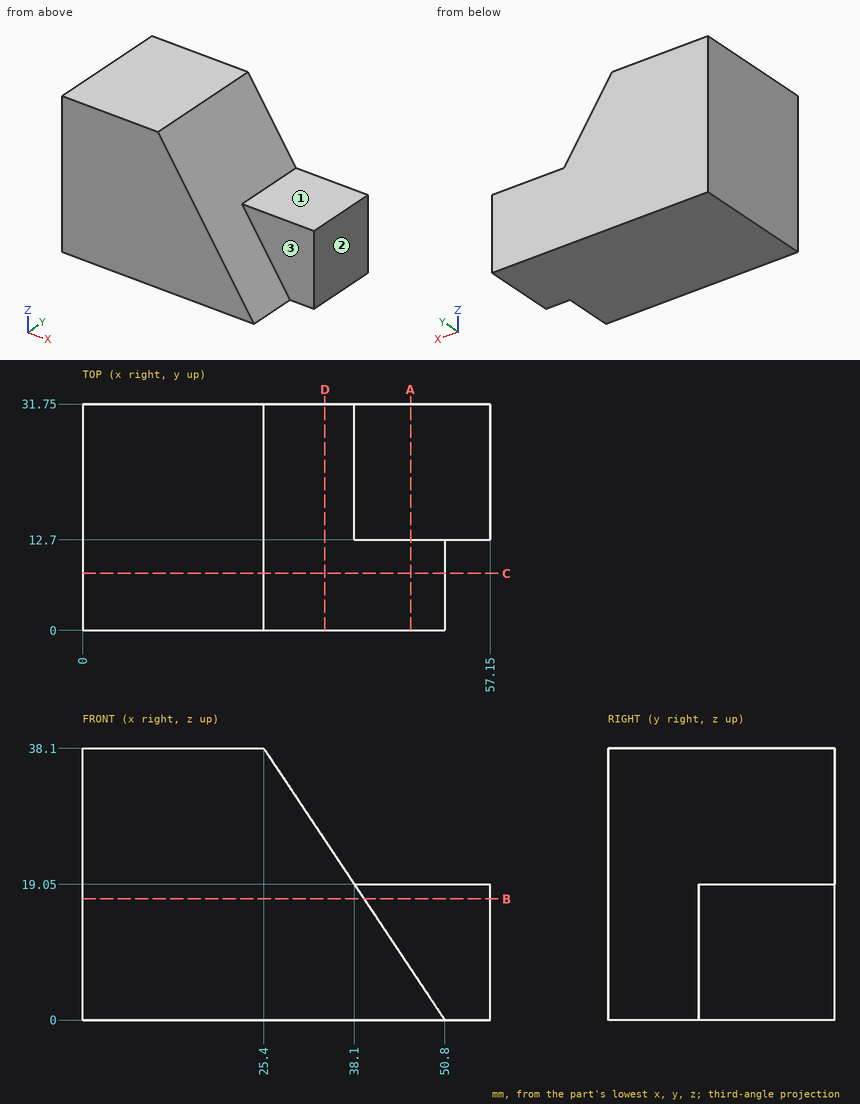
Here's the drawing with two shaded views (mm, measured from the low corner). I have some questions. A direction names the side the tool comes from. Coordinates: 2 decimals unless noted, no trailing zeros. Loops run counter-clockwise (first coordinate to the right, second up) from the corner with the lowest first, then second, coordinate; pieces in that order, holes last. Notation, with made-up numbers: M 50.25,-2 L 98.25,-2 A28 ccw 98.25,31 Z; hole C 6.25,82 d3. An arc over 180 degrees is marked long. Return JSON: item names as keys, results as strings. Group by question number.
Item 1: I'm going to push flat-ended pins straight in: pin 1 Ø5 at (y, z) = (19, 21) entering from +X; pin 2 Ø6 at (x, y) = (31, 22.5) entering from +Z; pin 3 Ø8 at (x, y) = (43, 20) entering from +Z; pin 4 Ø2 at (y, z) = (3.5, 30) entering from +X. Where does each tip first touch, or does it pass through?
Item 2: Imagine slicing it at B-B (z = 17). Please give me the cut outline in (x, y), and give its area (3 significant figures).
Item 3: Imagine slicing it at A-A (x = 46). Please give me the cut outline in (y, z), and give its area (3 significant figures).
Item 4: Imagine slicing it at D-D (x = 34). Please give me the cut outline in (y, z).
Item 5: On a 3-axis mill with a long thin cutter (end or side, diameter ignored), from which of +Z, -Z, +X, -X, +Y, -Y can I reach the whole of each face in a straight line? I mean the marked faces 1, 2 and 3. Say none if no direction works.
Item 6: Imagine slicing it at C-C (y = 8). Please give me the cut outline in (x, z), and give its area (3 significant figures).
Item 7: If I drill on L1, parallel to Y at x = 50, z = 5; L2, parallel to X at y = 8, z = 18.5; L3, parallel to Z at x = 33, y = 18.5, over which ranges is the centre line in solid material (lowest first)? Write a range as from..to.
Verdict:
{
 "1": {"pin 1": "stops at x = 57.15", "pin 2": "stops at z = 34.2", "pin 3": "stops at z = 19.05", "pin 4": "stops at x = 31.47"},
 "2": {"outline": "M 0,0 L 39.47,0 L 39.47,12.7 L 57.15,12.7 L 57.15,31.75 L 0,31.75 Z", "area": "1,590 mm^2"},
 "3": {"outline": "M 0,0 L 31.75,0 L 31.75,19.05 L 12.7,19.05 L 12.7,7.2 L 0,7.2 Z", "area": "454 mm^2"},
 "4": {"outline": "M 0,0 L 31.75,0 L 31.75,25.2 L 0,25.2 Z"},
 "5": {"face 1": "+Z, +X, +Y, -Y", "face 2": "+Z, -Z, +X, +Y, -Y", "face 3": "+Z, +X, -Y"},
 "6": {"outline": "M 0,0 L 50.8,0 L 25.4,38.1 L 0,38.1 Z", "area": "1,450 mm^2"},
 "7": {"L1": "y = 12.7..31.75", "L2": "x = 0..38.47", "L3": "z = 0..26.7"}
}
